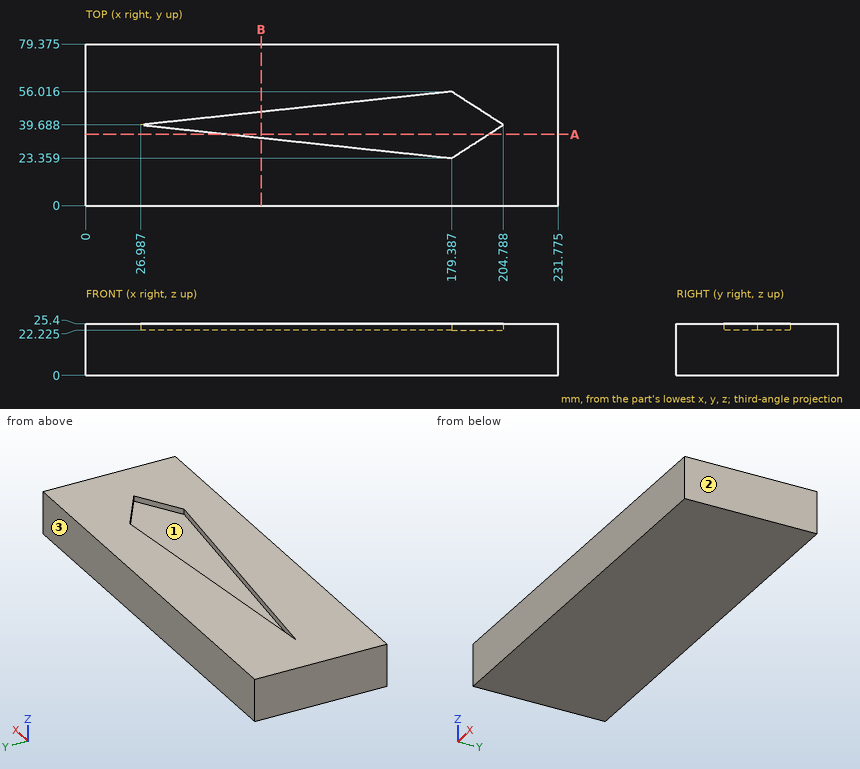
Could you check a few things on this drawing? It's one solid part, dimensions in mm from its lowest x, y, z. Give positions to 0.01 mm unless a question says otherwise; leave off trailing zeros. Write each loop counter-clockwise with the first axis right and the second up, starting at its lowest first coordinate (ties: lowest second). Pieces come first, ordered by that corner, then holes.
(1) Thinking about a two-plate mould opening in Y: for the marked faces 1, 2 and 3, which applies, pulls with the +Y half, pulls with the -Y half, needs draft (parallel to the pull), parting line crosses it, or undercut?
Output values:
face 1: undercut
face 2: needs draft
face 3: pulls with the +Y half
(2) If I drill on L1, parallel to Y at x = 151, z = 23.5 (1 decimal); L2, parallel to Z at x = 184.5, y = 31 (1 decimal), over which ranges is the centre line in solid material (lowest first)?
Output values:
L1: y = 0 to 26.4, 53 to 79.4
L2: z = 0 to 22.2
(3) Imagine slicing it at B-B, the plane x = 86. Write out the boundary of the cut face in (y, z) (1 decimal).
Output values:
outline: (0, 0) - (79.4, 0) - (79.4, 25.4) - (46, 25.4) - (46, 22.2) - (33.4, 22.2) - (33.4, 25.4) - (0, 25.4) - close
(4) Imagine slicing it at A-A, the plane y = 35. Write out the boundary of the cut face in (x, z) (1 decimal).
Output values:
outline: (0, 0) - (231.8, 0) - (231.8, 25.4) - (197.5, 25.4) - (197.5, 22.2) - (70.7, 22.2) - (70.7, 25.4) - (0, 25.4) - close
